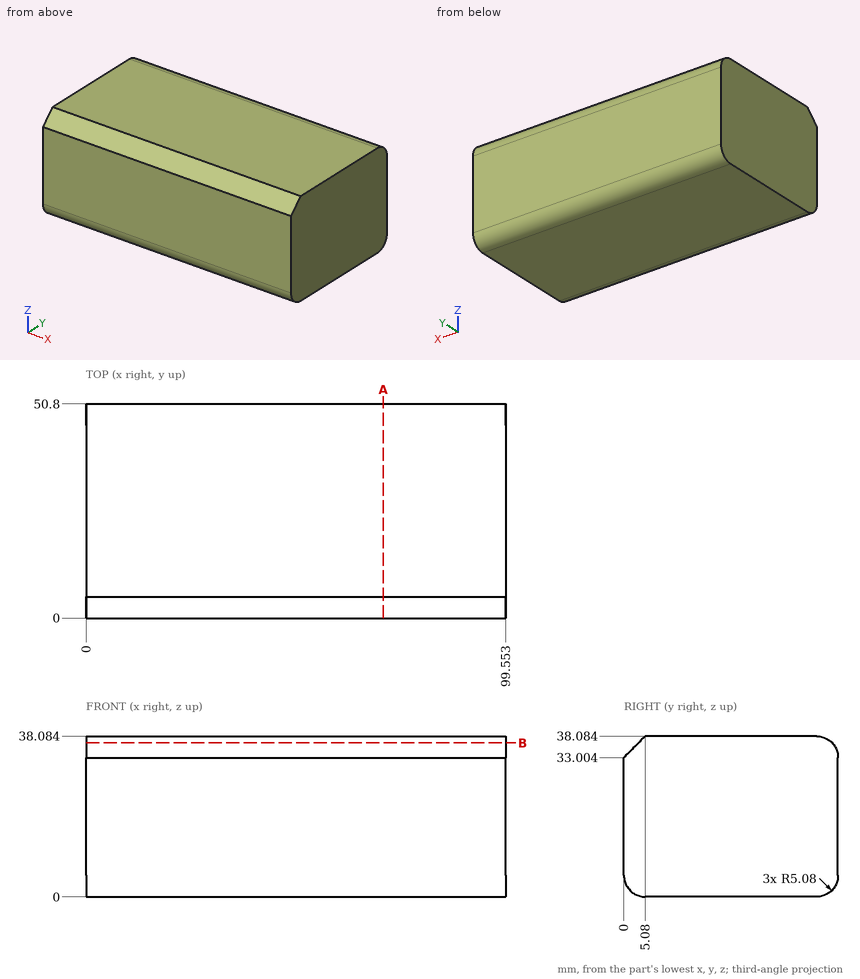
For this review, use the dimensioned drawing (mm, ordinates from the lowest corner) and the shaded views. Give positions to 0.01 mm unless a question says otherwise; leave off trailing zeros. Loops run counter-clockwise (first coordinate to the right, second up) from the corner with the lowest first, then second, coordinate; pieces in that order, holes last. Notation, with made-up numbers: (20, 53.5) - (67, 53.5) arc R21 ccw to (67, 81.5) - close; hole circle Ø7 at (28.25, 66). An arc over 180 degrees is marked (long way). Write each question's results on one line, items separated by ' | '.
(1) For line 1 along Z through (x, y) = (43, 47); line 2 along Y through (x, z) = (65, 2.5); line 3 along Z through (x, y) = (37, 4) (1 decimal), list the stretches that pass through material, from the lowest coordinate up.
Conclusion:
line 1: 0.16 to 37.92 | line 2: 0.7 to 50.1 | line 3: 0.1 to 37
(2) Take a section at A-A (x = 70.5). Give the boundary of the cut face in (y, z).
Conclusion:
outline: (0, 5.08) arc R5.08 ccw to (5.08, 0) - (45.72, 0) arc R5.08 ccw to (50.8, 5.08) - (50.8, 33) arc R5.08 ccw to (45.72, 38.08) - (5.08, 38.08) - (0, 33) - close
(3) Take a section at B-B (z = 36.5). Give the boundary of the cut face in (x, y), then the cut area to 3 significant figures.
Conclusion:
outline: (0, 3.5) - (99.55, 3.5) - (99.55, 49.41) - (0, 49.41) - close | area: 4,570 mm^2
(4) For pin 1 Ø6 at (x, z) = (40.5, 27) entering from -Y, flat-tipped, find the tip position at first contact; note if it passes through.
Conclusion:
pin 1: y = 0
